Build history of the part. All positions in model axes, mm. A direction names the side the tool comes from. Give positions to 0.01 mm unless a question says otherwise; leave off trailing zeros. Write each loop counter-clockwise with the first axis right and the second up, starting at its lowest first coordinate (ties: lowest second). Pieces come first, ordered by that corner, then holes.
from build123d import *

# Parameters (mm, degrees)
SKIZZE3_W                       = 20
SKIZZE3_H                       = 20
SKIZZE3_R                       = 7.5
AUFSATZ_LINEAR_AUSTRAGEN2_DEPTH = 5
SKIZZE4_R                       = 1.05
SCHNITT_LINEAR_AUSTRAGEN1_DEPTH = 6
SKIZZE5_R                       = 1.5
SCHNITT_LINEAR_AUSTRAGEN2_DEPTH = 2.5
SCHNITT_LINEAR_AUSTRAGEN3_DEPTH = 6
SKIZZE7_R                       = 1.15
SCHNITT_LINEAR_AUSTRAGEN4_DEPTH = 6
SKIZZE8_R                       = 2.5
SCHNITT_LINEAR_AUSTRAGEN5_DEPTH = 3


with BuildPart() as part:
    # Skizze2 → Rotation1 (revolve)
    with BuildSketch(Plane(origin=(0, 0, 0), x_dir=(0, 0, -1), z_dir=(1, 0, 0))):
        Polygon((0, 3.75), (-1, 3.75), (-1, 3.25), (-2.6, 3.25), (-2.6, 2), (-5, 2), (-5, 7.5), (0, 7.5), align=None)
    revolve(axis=Axis((0, 0, 12.6), (0, 0, -1)))

    # Skizze3 → Aufsatz-Linear austragen2 (add, through all)
    with BuildSketch(Plane.XY.offset(5)):
        Rectangle(SKIZZE3_W, SKIZZE3_H)
        Circle(SKIZZE3_R, mode=Mode.SUBTRACT)
    extrude(amount=-AUFSATZ_LINEAR_AUSTRAGEN2_DEPTH)

    # Skizze4 → Schnitt-Linear austragen1 (cut, through all)
    with BuildSketch(Plane.XY.offset(5)):
        with Locations((0, 5.5)):
            Circle(SKIZZE4_R)
        with Locations((0, -5.5)):
            Circle(SKIZZE4_R)
    extrude(amount=-SCHNITT_LINEAR_AUSTRAGEN1_DEPTH, mode=Mode.SUBTRACT)

    # Skizze5 → Schnitt-Linear austragen2 (cut)
    with BuildSketch(Plane.XY.offset(5)):
        with Locations((0, 5.5)):
            Circle(SKIZZE5_R)
        with Locations((0, -5.5)):
            Circle(SKIZZE5_R)
    extrude(amount=-SCHNITT_LINEAR_AUSTRAGEN2_DEPTH, mode=Mode.SUBTRACT)

    # Skizze6 → Schnitt-Linear austragen3 (cut, through all)
    with BuildSketch(Plane.XY.offset(5)):
        with BuildLine():
            Line((-10, 7.352290732), (-10.887824638, 7.352290732))
            Line((-10.887824638, 7.352290732), (-10.887824638, 10.887824638))
            Line((-10.887824638, 10.887824638), (-7.352290732, 10.887824638))
            Line((-7.352290732, 10.887824638), (-7.352290732, 10))
            ThreePointArc((-7.352290732, 10), (-9.22450391, 9.22450391), (-10, 7.352290732))
        make_face()
        with BuildLine():
            Line((7.352290732, 10.887824638), (7.352290732, 10))
            ThreePointArc((7.352290732, 10), (9.22450391, 9.22450391), (10, 7.352290732))
            Line((10, 7.352290732), (10.887824638, 7.352290732))
            Line((10.887824638, 7.352290732), (10.887824638, 10.887824638))
            Line((10.887824638, 10.887824638), (7.352290732, 10.887824638))
        make_face()
        with BuildLine():
            Line((10, -7.352290732), (10.887824638, -7.352290732))
            Line((10.887824638, -7.352290732), (10.887824638, -10.887824638))
            Line((10.887824638, -10.887824638), (7.352290732, -10.887824638))
            Line((7.352290732, -10.887824638), (7.352290732, -10))
            ThreePointArc((7.352290732, -10), (9.22450391, -9.22450391), (10, -7.352290732))
        make_face()
        with BuildLine():
            Line((-7.352290732, -10.887824638), (-7.352290732, -10))
            ThreePointArc((-7.352290732, -10), (-9.22450391, -9.22450391), (-10, -7.352290732))
            Line((-10, -7.352290732), (-10.887824638, -7.352290732))
            Line((-10.887824638, -7.352290732), (-10.887824638, -10.887824638))
            Line((-10.887824638, -10.887824638), (-7.352290732, -10.887824638))
        make_face()
    extrude(amount=-SCHNITT_LINEAR_AUSTRAGEN3_DEPTH, mode=Mode.SUBTRACT)

    # Skizze7 → Schnitt-Linear austragen4 (cut, through all)
    with BuildSketch(Plane.XY.offset(5)):
        with Locations((-7.352290732, 7.352290732)):
            Circle(SKIZZE7_R)
        with Locations((7.352290732, 7.352290732)):
            Circle(SKIZZE7_R)
        with Locations((7.352290732, -7.352290732)):
            Circle(SKIZZE7_R)
        with Locations((-7.352290732, -7.352290732)):
            Circle(SKIZZE7_R)
    extrude(amount=-SCHNITT_LINEAR_AUSTRAGEN4_DEPTH, mode=Mode.SUBTRACT)

    # Skizze8 → Schnitt-Linear austragen5 (cut)
    with BuildSketch(Plane.XY.offset(5)):
        with Locations((-7.352290732, 7.352290732)):
            Circle(SKIZZE8_R)
        with Locations((7.352290732, 7.352290732)):
            Circle(SKIZZE8_R)
        with Locations((7.352290732, -7.352290732)):
            Circle(SKIZZE8_R)
        with Locations((-7.352290732, -7.352290732)):
            Circle(SKIZZE8_R)
    extrude(amount=-SCHNITT_LINEAR_AUSTRAGEN5_DEPTH, mode=Mode.SUBTRACT)


solid = part.part
(1) Saw through at D-D, the plane x = -0.75. Give the number of separate pieces and of enclosed holes in the cut face, plus the area to 3 significant figures.
(2) 3-axis set-ups, long thin cutter, end or side, ignore diameter. For faces 5 (the face through (-9.19, -5.66, 3.52)), 6 (the face through (-0.14, 6.54, 1.27)): which of +Z, -Z, +X, -X, +Y, -Y reach the whole face in a straight line?
(3) Drop flat-ended pins along their axis: pin 1 (1.5 mm diameter, centred on x = -8, y = 6.5, fed in from +Z); pin 2 (4 mm diameter, centred on x = -1, y = 0.5, fed in from -Z). Give the stop position or say it passes through.
(4) Saw through at A-A, the plane z = 3.9. List the corners of the cut face in (x, y), plus the area to 3 significant figures.
(5) Mould opens along Y. For faces 1 (the face through (-6.29, -7.79, 1.01)), 2 (the face through (0, 10, 3)), 3 (the face through (-0.1, 2.4, 5)), 4 (the face through (0, -10, 3)) say: +Y half, -Y half, draft (parallel to the pull), parting line (faces both ways), or undercut.
(6) Saw through at C-C, the plane y = 0. List the corners of the cut face in (x, z), plus the area to 3 significant figures.
(7) Saw through at B-B, the plane x = 1.75. List the corners of the cut face in (y, z).
(8) Probe line 1 (X direction, y = 0, z = 1.6); line 2 (X direction, y = 8, z = 1.75); line 3 (X direction, y = 0, z = 3.7). List the from-to ranges inside material, lowest first.
Computed values:
1. separate pieces: 4
1. enclosed holes: 0
1. area: 53.3 mm2
2. face 5: +Z
2. face 6: +Z, -Z
3. pin 1: stops at z = 2
3. pin 2: stops at z = 2.6
4. outline: (-10, -7.35) arc R2.65 ccw to (-7.35, -10) - (7.35, -10) arc R2.65 ccw to (10, -7.35) - (10, 7.35) arc R2.65 ccw to (7.35, 10) - (-7.35, 10) arc R2.65 ccw to (-10, 7.35) - close; hole circle Ø5 at (-7.35, -7.35); hole circle Ø5 at (-7.35, 7.35); hole circle Ø4 at (0, 0); hole circle Ø3 at (0, -5.5); hole circle Ø3 at (0, 5.5); hole circle Ø5 at (7.35, -7.35); hole circle Ø5 at (7.35, 7.35)
4. area: 289 mm2
5. face 1: undercut
5. face 2: +Y half
5. face 3: draft
5. face 4: -Y half
6. outline: (-10, 0) - (-3.75, 0) - (-3.75, 1) - (-3.25, 1) - (-3.25, 2.6) - (-2, 2.6) - (-2, 5) - (-10, 5) - close; (2, 2.6) - (3.25, 2.6) - (3.25, 1) - (3.75, 1) - (3.75, 0) - (10, 0) - (10, 5) - (2, 5) - close
6. area: 72.5 mm2
7. outline: (-10, 0) - (-3.32, 0) - (-3.32, 1) - (-2.74, 1) - (-2.74, 2.6) - (-0.97, 2.6) - (-0.97, 5) - (-10, 5) - close; (0.97, 2.6) - (2.74, 2.6) - (2.74, 1) - (3.32, 1) - (3.32, 0) - (10, 0) - (10, 5) - (0.97, 5) - close
8. line 1: x = -10 to -3.25, 3.25 to 10
8. line 2: x = -9.92 to -8.3, -6.4 to 6.4, 8.3 to 9.92
8. line 3: x = -10 to -2, 2 to 10
